Here's how the part is built. I have some questions about the finished solid (model axes, mm). A direction names the side the tool comes from. Give positions to 0.01 mm unless a question says otherwise; leave off trailing zeros. Write each loop counter-clockwise with the first axis right and the second up, starting at its lowest first coordinate (ties: lowest second). Pieces come first, ordered by that corner, then holes. Notation, with made-up numbers: (-1.5, -24) - (33.5, -24) arc R23 cw to (33.5, -1) - close; hole circle Ø10 at (-26, 47). An arc over 180 degrees is marked (long way). Use a Markdown table: item, result.
```python
from build123d import *

# Parameters (mm, degrees)
BASE_DEPTH         = 5
BASE_DEPTH_BACK    = 5
ESQUISSE1_R        = 2
ESQUISSE2_W        = 75
ESQUISSE2_H        = 5
BOSS_GRAND_DEPTH   = 10
ESQUISSE3_W        = 75
ESQUISSE3_H        = 5
BOSS_PETIT_DEPTH   = 10
ESQUISSE4_W        = 5
ESQUISSE4_H        = 15
BLOQUER_DEPTH      = 5
ESQUISSE5_W        = 5
ESQUISSE5_H        = 15
VIDE_BLOQUER_DEPTH = 5
ESQUISSE6_W        = 80
ESQUISSE6_H        = 5
BOSSE_BAS_DEPTH    = 10
ESQUISSE7_R        = 2
BOSS_EXTRU_6_DEPTH = 5


with BuildPart() as part:
    # Esquisse1 → BASE (new, two sides: drawn at the far end of the back side and taken through both)
    with BuildSketch(Plane.XY.offset(-BASE_DEPTH_BACK)):
        with BuildLine():
            Line((-80, 2.5), (0, 2.5))
            Line((0, 2.5), (0, -2.5))
            Line((0, -2.5), (-80, -2.5))
            ThreePointArc((-80, -2.5), (-82.5, 0), (-80, 2.5))
        make_face()
        with Locations((-80, 0)):
            Circle(ESQUISSE1_R, mode=Mode.SUBTRACT)
    extrude(amount=BASE_DEPTH + BASE_DEPTH_BACK)

    # Esquisse2 → BOSS GRAND (add)
    with BuildSketch(Plane.XY.offset(5)):
        with Locations((-37.5, 0)):
            Rectangle(ESQUISSE2_W, ESQUISSE2_H)
    extrude(amount=BOSS_GRAND_DEPTH)

    # Esquisse3 → BOSS PETIT (add)
    with BuildSketch(Plane(origin=(0, 0, -5), x_dir=(-1, 0, 0), z_dir=(0, 0, -1))):
        with Locations((37.5, 0)):
            Rectangle(ESQUISSE3_W, ESQUISSE3_H)
    extrude(amount=BOSS_PETIT_DEPTH)

    # Esquisse4 → BLOQUER (add)
    with BuildSketch(Plane(origin=(0, 2.5, 0), x_dir=(1, 0, 0), z_dir=(0, 1, 0))):
        with Locations((2.5, 7.5)):
            Rectangle(ESQUISSE4_W, ESQUISSE4_H)
    extrude(amount=-BLOQUER_DEPTH)

    # Esquisse5 → VIDE BLOQUER (cut)
    with BuildSketch(Plane(origin=(0, 2.5, 0), x_dir=(1, 0, 0), z_dir=(0, 1, 0))):
        with Locations((-2.5, -7.5)):
            Rectangle(ESQUISSE5_W, ESQUISSE5_H)
    extrude(amount=-VIDE_BLOQUER_DEPTH, mode=Mode.SUBTRACT)

    # Esquisse6 → BOSSE BAS (add)
    with BuildSketch(Plane.XY.offset(15)):
        with Locations((-35, 0)):
            Rectangle(ESQUISSE6_W, ESQUISSE6_H)
    extrude(amount=BOSSE_BAS_DEPTH)

    # Esquisse7 → Boss.-Extru.6 (add)
    with BuildSketch(Plane.XZ.offset(2.5)):
        with Locations(Location((-10, -10, 0), (0, 0, 270))):
            Circle(ESQUISSE7_R)
    extrude(amount=BOSS_EXTRU_6_DEPTH)


solid = part.part
```
Item 1: If we section it at B-B, the plane x = -2: Write out the boundary of the cut face in (y, z).
Values:
| item | result |
|---|---|
| outline | (-2.5, -15) - (2.5, -15) - (2.5, 0) - (-2.5, 0) - close; (-2.5, 15) - (2.5, 15) - (2.5, 25) - (-2.5, 25) - close |
Item 2: Will these pins go through, and if not, where does the flat tip stop? pin 1 Ø2 at (x, z) = (-24, -5) entering from -Y; pin 2 Ø2.5 at (x, y) = (-80, 0) entering from +Z; pin 3 Ø2.5 at (y, z) = (1, 12.5) entering from -X; pin 4 Ø2.5 at (y, z) = (0.5, 7) entering from +X.
Values:
| item | result |
|---|---|
| pin 1 | stops at y = -2.5 |
| pin 2 | passes through |
| pin 3 | stops at x = -75 |
| pin 4 | stops at x = -5 |
Item 3: Thinking about a two-plate mould opening in Z: for faces 1 (the flat face through (-36, 0, 25)), 2 (the flat face through (-5, 0, 8)), 3 (the flat face through (-78, -1, -5)), 4 (the flat face through (-75, 0, 15)), which applies, +Z half, -Z half, draft (parallel to the pull), parting line (faces both ways), or undercut?
Values:
| item | result |
|---|---|
| face 1 | +Z half |
| face 2 | undercut |
| face 3 | -Z half |
| face 4 | draft |
Item 4: If we section it at D-D, the plane z = -10: Write out the boundary of the cut face in (x, y).
Values:
| item | result |
|---|---|
| outline | (-75, -2.5) - (-12, -2.5) - (-12, -7.5) - (-8, -7.5) - (-8, -2.5) - (5, -2.5) - (5, 2.5) - (-75, 2.5) - close |
Item 5: If we section it at C-C, the plane z = -3: Write out the boundary of the cut face in (x, y).
Values:
| item | result |
|---|---|
| outline | (-80, -2.5) - (5, -2.5) - (5, 2.5) - (-80, 2.5) arc R2.5 ccw to start; hole circle Ø4 at (-80, 0) |
Item 6: For faces 5 (the flat face through (-78, -1, 5)), 6 (the flat face through (0, 0, 0)), 7 (the cylindrical face through (-78.092, 0.601, -0.07)), 8 (the flat face through (-75, 0, -10)), 9 (the cylindrical face through (-8, -5, -10)), which set-ups out of +Z, -Z, +X, -X, +Y, -Y let a thin tool reach every point of the face, with its end or its side?
Values:
| item | result |
|---|---|
| face 5 | +Z, -X, +Y, -Y |
| face 6 | +X, +Y, -Y |
| face 7 | +Z, -Z |
| face 8 | -Z, -X, +Y, -Y |
| face 9 | -Y |
Item 7: I need wall thicknesses on line 1 along Z through (x, y) = (-0.5, -1.5); line 2 along Y through (x, z) = (-80, 1.5); line 3 along Y through (x, z) = (-42.5, -7). Which ranges of each line are inside material? Lowest first, please. Write a range as [from, to].
Values:
| item | result |
|---|---|
| line 1 | z = [-15, 0], [15, 25] |
| line 2 | y = [-2.5, -2], [2, 2.5] |
| line 3 | y = [-2.5, 2.5] |
Item 8: If we section it at A-A, the plane y = 0: Write out the boundary of the cut face in (x, z).
Values:
| item | result |
|---|---|
| outline | (-82.5, -5) - (-82, -5) - (-82, 5) - (-82.5, 5) - close; (-78, -5) - (-75, -5) - (-75, -15) - (5, -15) - (5, 0) - (-5, 0) - (-5, 15) - (5, 15) - (5, 25) - (-75, 25) - (-75, 5) - (-78, 5) - close |
